```python
from build123d import *

# Parameters (mm, degrees)
BOSS_EXTRUDE1_DEPTH  = 25
CUT_EXTRUDE1_DEPTH   = 39.494845434
M4_CLEARANCE_HOLE1_D = 4.5
SKETCH5_W            = 25.4
SKETCH5_H            = 3.175
BOSS_EXTRUDE2_DEPTH  = 20
SKETCH6_W            = 25.4
SKETCH6_H            = 3.175
BOSS_EXTRUDE3_DEPTH  = 20
M4_CLEARANCE_HOLE2_D = 4.5
CUT_EXTRUDE2_DEPTH   = 55.05715147
FILLET1_R            = 3


with BuildPart() as part:
    # Sketch1 → Boss-Extrude1 (new, symmetric)
    with BuildSketch(Plane(origin=(0, 0, 0), x_dir=(0, 0, -1), z_dir=(1, 0, 0))):
        Polygon((0, 0), (0, -19.05), (25.4, -19.05), (25.4, -15.875), (3.175, -15.875), (3.175, 0), align=None)
    extrude(amount=BOSS_EXTRUDE1_DEPTH, both=True)

    # Sketch2 → Cut-Extrude1 (cut, through all)
    with BuildSketch(Plane(origin=(0, 0, -3.175), x_dir=(-1, 0, 0), z_dir=(0, 0, -1))):
        Polygon((-25, -15.875), (-9.125, 0), (-25, 0), align=None)
        Polygon((25, -15.875), (9.125, 0), (25, 0), align=None)
    extrude(amount=-CUT_EXTRUDE1_DEPTH, mode=Mode.SUBTRACT)

    # M4 Clearance Hole1 (through all)
    with Locations(Plane(origin=(0, 0, -3.175), x_dir=(-1, 0, 0), z_dir=(0, 0, -1))):
        with Locations((-12.7, -11.4453125), (12.7, -11.4453125)):
            Hole(M4_CLEARANCE_HOLE1_D / 2)

    # Sketch5 → Boss-Extrude2 (add)
    with BuildSketch(Plane(origin=(25, 0, 0), x_dir=(0, 0, -1), z_dir=(1, 0, 0))):
        with Locations((12.7, -17.4625)):
            Rectangle(SKETCH5_W, SKETCH5_H)
    extrude(amount=BOSS_EXTRUDE2_DEPTH)

    # Sketch6 → Boss-Extrude3 (add)
    with BuildSketch(Plane.ZY.offset(25)):
        with Locations((-12.7, -17.4625)):
            Rectangle(SKETCH6_W, SKETCH6_H)
    extrude(amount=BOSS_EXTRUDE3_DEPTH)

    # M4 Clearance Hole2 (through all)
    with Locations(Plane(origin=(0, -15.875, 0), x_dir=(1, 0, 0), z_dir=(0, 1, 0))):
        with Locations((37.5, 12.5), (-37.5, 12.5)):
            Hole(M4_CLEARANCE_HOLE2_D / 2)

    # Sketch9 → Cut-Extrude2 (cut, through all)
    with BuildSketch(Plane(origin=(0, -15.875, 0), x_dir=(1, 0, 0), z_dir=(0, 1, 0))):
        Polygon((40.5, 25.4), (-40.5, 25.4), (-32.5, 12.4), (32.5, 12.4), align=None)
    extrude(amount=-CUT_EXTRUDE2_DEPTH, mode=Mode.SUBTRACT)

    # Fillet1
    # the kernel refuses this fillet: 3 mm, written as the material it takes off along each edge
    with BuildSketch(Plane(origin=(-45, -26.55, -25.4), x_dir=(0, 0, 1), z_dir=(0, 1, 0)), Plane(origin=(45, -8.375, -25.4), x_dir=(0, 0, 1), z_dir=(0, -1, 0))) as fillet1_piece_1:
        with BuildLine():
            CenterArc((FILLET1_R, FILLET1_R), FILLET1_R, 180, 90)
            Line((0, FILLET1_R), (0, 0))
            Line((0, 0), (FILLET1_R, 0))
        make_face()
    extrude(amount=18.175, mode=Mode.SUBTRACT)
    with BuildSketch(Plane(origin=(-40.5, -11.684036045, -25.4), x_dir=(-1, 0, 0), z_dir=(0, -1, 0)), Plane(origin=(40.5, -11.684036045, -25.4), x_dir=(-0.5240974256643328, 0, 0.8516583167045451), z_dir=(0, -1, 0))) as fillet1_piece_2:
        with BuildLine():
            CenterArc((FILLET1_R * 0.558795194036, -FILLET1_R), FILLET1_R, 90, 58.392497754)
            Line((-FILLET1_R * 0.292863122668, -FILLET1_R * 0.475902574336), (0, 0))
            Line((0, 0), (FILLET1_R * 0.558795194036, 0))
        make_face()
    extrude(amount=11.556927911, mode=Mode.SUBTRACT)
    with BuildSketch(Plane(origin=(45, -26.55, 0), x_dir=(-1, 0, 0), z_dir=(0, 1, 0)), Plane(origin=(-45, -8.375, 0), x_dir=(1, 0, 0), z_dir=(0, -1, 0))) as fillet1_piece_3:
        with BuildLine():
            CenterArc((FILLET1_R, -FILLET1_R), FILLET1_R, 90, 90)
            Line((0, -FILLET1_R), (0, 0))
            Line((0, 0), (FILLET1_R, 0))
        make_face()
    extrude(amount=18.175, mode=Mode.SUBTRACT)


solid = part.part
```
Geometry check sheet. Reference: the model listing, model coordinates, mm. A direction names the side the tool comes from. Give positions to 0.01 mm unless a question says otherwise; leave off trailing zeros. Write each loop counter-clockwise with the first axis right and the second up, starting at its lowest first coordinate (ties: lowest second). Pieces come first, ordered by that corner, then holes. Notation, with made-up numbers: (49.5, 65) -> (72.5, 65) arc R19 cw to (72.5, 96) -> close; hole circle Ø10 at (46.25, 6.25). An arc over 180 degrees is marked (long way). One line per question, with ' | ' between items.
Item 1: Depth check by flat-ended pin: pin 1 (5 mm diameter, centred on x = 6, y = -6.5, fed in from -Z) (3 decimals); pin 2 (2.5 mm diameter, centred on x = -11, y = -17, fed in from -Z); pin 3 (6 mm diameter, centred on x = 37.5, z = -12.5, fed in from +Y) (3 decimals). Enter the tip coordinate at first touch or a pass-through.
Determined:
pin 1: z = -3.175 | pin 2: z = -12.4 | pin 3: y = -15.875
Item 2: Sectioned sample at C-C, the plane x = -12.7. Record the boundary of the cut face in (y, z) (3 decimals).
Determined:
outline: (-19.05, -12.4) -> (-15.875, -12.4) -> (-15.875, -3.175) -> (-13.695, -3.175) -> (-13.695, 0) -> (-19.05, 0) -> close; (-9.195, -3.175) -> (-3.575, -3.175) -> (-3.575, 0) -> (-9.195, 0) -> close
Item 3: Draft check along Z on faces 1 (the flat face through (1, -12, 0)), 2 (the cylindrical face through (-38.71, -17.485, -14.397)), 3 (the flat face through (-36.11, -17.44, -18.27)), 4 (the flat face through (45, -17, -13)). Enter one of: released by +Z, released by -Z, zero draft, split by the parting line, or undercut.
Determined:
face 1: released by +Z | face 2: undercut | face 3: released by -Z | face 4: zero draft
Item 4: Sectioned sample at B-B, the plane z = -13.5. Record the boundary of the cut face in (x, y) (3 decimals), plus the area to 3 significant figures.
Determined:
outline: (-45, -19.05) -> (-39.516, -19.05) -> (-39.516, -15.875) -> (-45, -15.875) -> close; (-35.484, -19.05) -> (-33.177, -19.05) -> (-33.177, -15.875) -> (-35.484, -15.875) -> close; (33.177, -19.05) -> (35.484, -19.05) -> (35.484, -15.875) -> (33.177, -15.875) -> close; (39.516, -19.05) -> (45, -19.05) -> (45, -15.875) -> (39.516, -15.875) -> close | area: 49.5 mm^2
Item 5: Access from +Z, -Z, +X, -X, +Y, -Y to the whole of each face (thin tool, end or side, straight path). Record for faces 5 (the cylindrical face through (44.1, -17.48, -0.86)), 6 (the cylindrical face through (40.66, -17.44, -24.99)).
Determined:
face 5: +Z, +X, +Y, -Y | face 6: -Z, +Y, -Y
Item 6: Sectioned sample at A-A, the plane y = -18. Record the boundary of the cut face in (x, z).
Determined:
outline: (-45, -22.4) arc R3 ccw to (-42.09, -25.4) arc R3 ccw to (-39.62, -23.97) -> (-32.5, -12.4) -> (32.5, -12.4) -> (39.62, -23.97) arc R3 ccw to (42.09, -25.4) arc R3 ccw to (45, -22.4) -> (45, -3) arc R3 ccw to (42, 0) -> (-42, 0) arc R3 ccw to (-45, -3) -> close; hole circle Ø4.5 at (-37.5, -12.5); hole circle Ø4.5 at (37.5, -12.5)
Item 7: Sectioned sample at D-D, the plane x = 7. Record the boundary of the cut face in (y, z) (3 decimals), plus the area to 3 significant figures.
Determined:
outline: (-19.05, -12.4) -> (-15.875, -12.4) -> (-15.875, -3.175) -> (0, -3.175) -> (0, 0) -> (-19.05, 0) -> close | area: 89.8 mm^2
Item 8: Scan lines: line 1 along X through (y, z) = (-17.9, -12.5); line 2 along X through (y, z) = (-17.25, -13.75); line 3 along Y through (x, z) = (32.5, -9) (3 decimals). Record each from-to range of solid material in increasing order.
Determined:
line 1: -45 to -39.75, -35.25 to -32.56, 32.56 to 35.25, 39.75 to 45 | line 2: -45 to -39.37, -35.63 to -33.33, 33.33 to 35.63, 39.37 to 45 | line 3: -19.05 to -15.875
